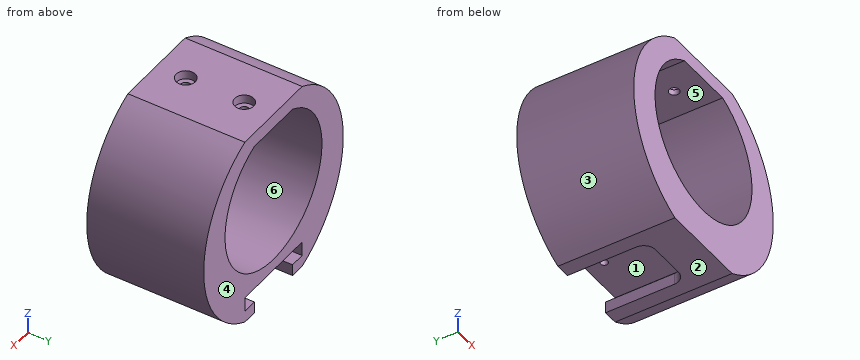
from build123d import *

# Parameters (mm, degrees)
BOSS_EXTRUDE1_DEPTH            = 20
CUT_EXTRUDE1_DEPTH             = 27.5
FILLET1_R                      = 4
CBORE_FOR_M3_SHCS1_D           = 3.4
CBORE_FOR_M3_SHCS1_DEPTH       = 5
CBORE_FOR_M3_SHCS1_CBORE_D     = 6.5
CBORE_FOR_M3_SHCS1_CBORE_DEPTH = 3
M3X0_5_TAPPED_HOLE1_D          = 2.5
M3X0_5_TAPPED_HOLE1_DEPTH      = 11
M3X0_5_TAPPED_HOLE1_TIP        = 0.751075774


with BuildPart() as part:
    # Sketch1 → Boss-Extrude1 (new body, symmetric)
    with BuildSketch(Plane(origin=(0, 0, 0), x_dir=(1, 0, 0), z_dir=(0, 1, 0))):
        with BuildLine():
            Line((-15, -28.348661632), (15, -28.348661632))
            ThreePointArc((15, -28.348661632), (36.566832412, 5), (15, 38.348661632))
            Line((15, 38.348661632), (-15, 38.348661632))
            ThreePointArc((-15, 38.348661632), (-36.566832412, 5), (-15, -28.348661632))
        make_face()
        with BuildLine():
            Line((-10, -23.348661632), (10, -23.348661632))
            ThreePointArc((10, -23.348661632), (0, 25.4), (-10, -23.348661632))
        make_face(mode=Mode.SUBTRACT)
    extrude(amount=BOSS_EXTRUDE1_DEPTH, both=True)

    # Sketch3 → Cut-Extrude1 (cut)
    with BuildSketch(Plane(origin=(0, 20, 0), x_dir=(1, 0, 0), z_dir=(0, 1, 0))):
        Polygon((-10, 38.348661632), (-10, 34.348661632), (-15, 34.348661632), (-15, 29.348661632), (15, 29.348661632), (15, 34.348661632), (10, 34.348661632), (10, 38.348661632), align=None)
    extrude(amount=-CUT_EXTRUDE1_DEPTH, mode=Mode.SUBTRACT)

    # Fillet1
    fillet1_edges = [part.edges().sort_by_distance(p)[0] for p in [
        (10, -7.5, -36.348661632),
        (15, -7.5, -31.848661632),
        (-15, -7.5, -31.848661632),
        (-10, -7.5, -36.348661632),
    ]]
    fillet(fillet1_edges, radius=FILLET1_R)

    # CBORE for M3 SHCS1
    with Locations(Plane.XY.offset(28.348661632)):
        with Locations((0, 10), (0, -10)):
            CounterBoreHole(CBORE_FOR_M3_SHCS1_D / 2, CBORE_FOR_M3_SHCS1_CBORE_D / 2, CBORE_FOR_M3_SHCS1_CBORE_DEPTH, depth=CBORE_FOR_M3_SHCS1_DEPTH)

    # M3x0.5 Tapped Hole1
    with Locations(Plane(origin=(0, 0, -38.348661632), x_dir=(-1, 0, 0), z_dir=(0, 0, -1))):
        with Locations((0, 13.90875121)):
            Hole(M3X0_5_TAPPED_HOLE1_D / 2, depth=M3X0_5_TAPPED_HOLE1_DEPTH)
            with Locations((0, 0, -(M3X0_5_TAPPED_HOLE1_DEPTH + M3X0_5_TAPPED_HOLE1_TIP / 2))):  # 118° drill point
                Cone(0, M3X0_5_TAPPED_HOLE1_D / 2, M3X0_5_TAPPED_HOLE1_TIP, mode=Mode.SUBTRACT)


solid = part.part
Geometry check sheet. Reference: the model listing, model coordinates, mm. Face numbers are marked on the shaded views. A direction names the side the tool comes from. Coordinates: 2 decimals unless noted, no trailing zeros. Order: outer loops, then holes, each group sorted by start corner. A loop starts at its lowest first (then second) coordinate and runs counter-clockwise, first axis right, second up. Notation, with made-up numbers: (-12.75, 82) - (-8.75, 82) arc R19 ccw to (-8.75, 115) - close; hole circle Ø7 at (21.5, 65). An arc over 180 degrees is marked (long way). Answer in a Markdown table with one row per item. Add a question column.
1) Cross-section at B-B, the plane x = 19. Record the cut outline in (y, z), then the cut area to 3 significant figures.
2) Cross-section at C-C, the plane z = 0. Record the cut outline in (x, y), then the cut area to 3 significant figures.
3) Cross-section at D-D, the plane y = 10. Record the cut outline in (x, z).
4) Gauge pin test, flat ends, axial feed: P1, Ø6, axis at x = 23, y = 14.5, coming from the -Z side; P2, Ø4, axis at y = 7.5, z = -32.5, coming from the -X side; P3, Ø7, axis at x = 1.5, z = -33.5, coming from the +Y side; P4, Ø8.5, axis at x = 0, y = 10, coming from the +Z side. Record the tip position at first contact, or that the pin passes through.
5) Release check for a two-part mould opening along Z. For the marked faces 3, 4, 5 and 6 record: +Z half, -Z half, draft (parallel to the pull), parting line (faces both ways), or undercut.
6) Cross-section at A-A, the plane y = 5. Record the cut outline in (x, z), then the cut area to 3 significant figures.
7) Set-up check for the marked faces 1 and 2: record each of +Z, -Z, +X, -X, +Y, -Y from which the full face is reachable in a straight line by a thin tool's end or side.
8) Material ranges on line 1 along Y through (x, z) = (0, 26.95); line 2 along Y through (x, z) = (0, 24.65); line 3 along X through (y, z) = (1, -11.5), recorded low to high. Write a range as [from, to].
Check result:
| question | item | result |
|---|---|---|
| 1 | outline | (-20, -36.24) - (20, -36.24) - (20, -16.86) - (-20, -16.86) - close; (-20, 16.86) - (20, 16.86) - (20, 26.24) - (-20, 26.24) - close |
| 1 | area | 1,150 mm² |
| 2 | outline | (-36.22, -20) - (-25.4, -20) - (-25.4, 20) - (-36.22, 20) - close; (25.4, -20) - (36.22, -20) - (36.22, 20) - (25.4, 20) - close |
| 2 | area | 866 mm² |
| 3 | outline | (-15, -38.35) - (-10, -38.35) - (-10, -34.35) - (-15, -34.35) - (-15, -29.35) - (15, -29.35) - (15, -34.35) - (10, -34.35) - (10, -38.35) - (15, -38.35) arc R36.57 ccw to (15, 28.35) - (3.25, 28.35) - (3.25, 25.35) - (1.7, 25.35) - (1.7, 23.35) - (10, 23.35) arc R25.4 cw (long way) to (-10, 23.35) - (-1.7, 23.35) - (-1.7, 25.35) - (-3.25, 25.35) - (-3.25, 28.35) - (-15, 28.35) arc R36.57 ccw to start |
| 4 | P1 | stops at z = -35.61 |
| 4 | P2 | stops at x = -26.21 |
| 4 | P3 | stops at y = -7.5 |
| 4 | P4 | stops at z = 28.35 |
| 5 | face 3 | parting line |
| 5 | face 4 | draft |
| 5 | face 5 | undercut |
| 5 | face 6 | undercut |
| 6 | outline | (-15, -38.35) - (-10, -38.35) - (-10, -34.35) - (-15, -34.35) - (-15, -29.35) - (15, -29.35) - (15, -34.35) - (10, -34.35) - (10, -38.35) - (15, -38.35) arc R36.57 ccw to (15, 28.35) - (-15, 28.35) arc R36.57 ccw to start; hole (-10, 23.35) arc R25.4 ccw (long way) to (10, 23.35) - close |
| 6 | area | 1,840 mm² |
| 7 | face 1 | +Y |
| 7 | face 2 | -Z, +X, -X, +Y, -Y |
| 8 | line 1 | y = [-20, -13.25], [-6.75, 6.75], [13.25, 20] |
| 8 | line 2 | y = [-20, -11.7], [-8.3, 8.3], [11.7, 20] |
| 8 | line 3 | x = [-35.98, -22.65], [22.65, 35.98] |
